Source: three-view drawing plus pictorial views. Frame: mm from the lowest corner of the part. A direction names the side the tool comes from. Coordinates: 2 decimals unless noted, no trailing zeros. Write each loop counter-clockwise with the first axis right and the second up, starting at its lowest first coordinate (ties: lowest second). Pieces come first, ordered by that corner, then holes. Notation, with made-up numbers: (69.25, 77.5) -> (73.25, 77.5) arc R22 ccw to (73.25, 91.5) -> close; hole circle Ø3 at (73, 22.25). An arc over 180 degrees is marked (long way). Write item = value, one per line.
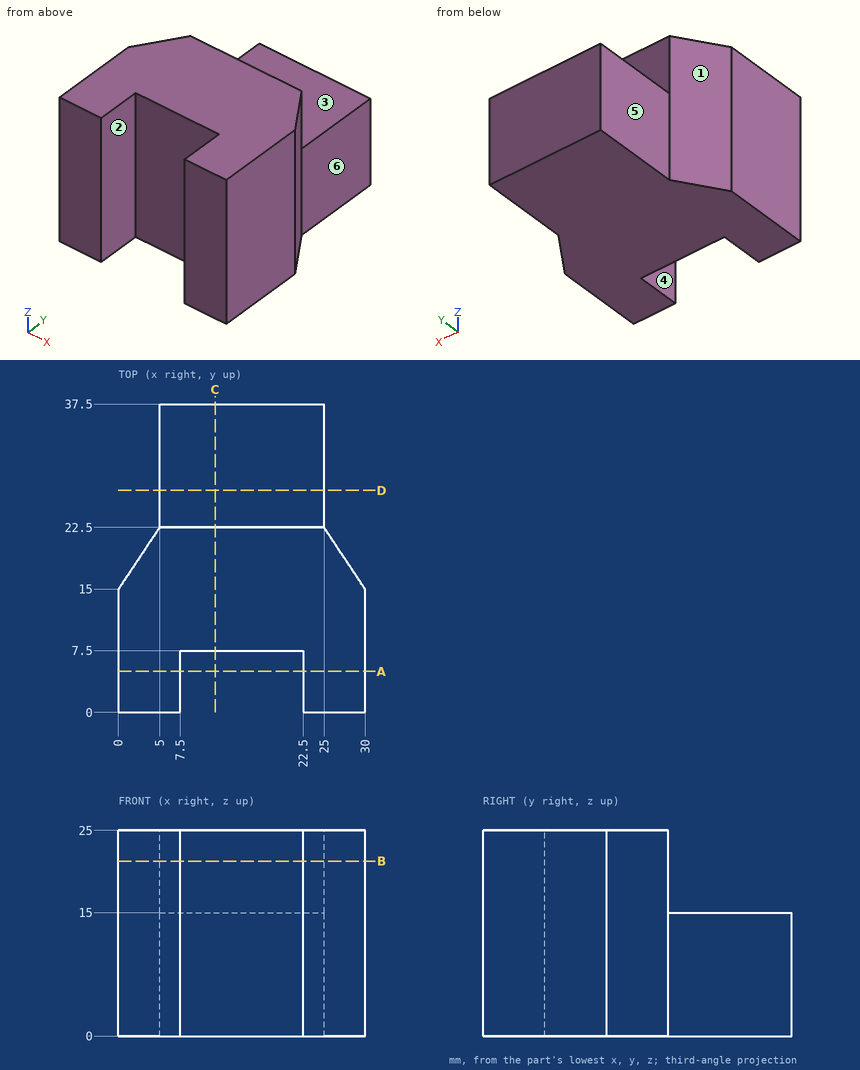
1) Cut plane B-B, the plane z = 21.25. Output: boundary loops of the cut face in (x, y).
Answer block:
outline = (0, 0) -> (7.5, 0) -> (7.5, 7.5) -> (22.5, 7.5) -> (22.5, 0) -> (30, 0) -> (30, 15) -> (25, 22.5) -> (5, 22.5) -> (0, 15) -> close
2) Cut plane C-C, the plane x = 11.75. Output: boundary loops of the cut face in (y, z), and give its area (3 significant figures).
Answer block:
outline = (7.5, 0) -> (37.5, 0) -> (37.5, 15) -> (22.5, 15) -> (22.5, 25) -> (7.5, 25) -> close
area = 600 mm2
3) First-contact query: pin 1 Ø6 at (x, z) = (16.5, 16) entering from -Y; pin 2 Ø7.5 at (y, z) = (30, 10) entering from +X; pin 3 Ø4.5 at (x, y) = (12.5, 31.5) entering from +Z. Flat tips, straight axial feed; report the tip coordinate or a pass-through.
Answer block:
pin_1 = 7.5
pin_2 = 25
pin_3 = 15
4) Cut plane D-D, the plane y = 27. Output: boundary loops of the cut face in (x, z).
Answer block:
outline = (5, 0) -> (25, 0) -> (25, 15) -> (5, 15) -> close
5) Cut plane A-A, the plane y = 5. Output: boundary loops of the cut face in (x, z).
Answer block:
outline = (0, 0) -> (7.5, 0) -> (7.5, 25) -> (0, 25) -> close; (22.5, 0) -> (30, 0) -> (30, 25) -> (22.5, 25) -> close
6) Pull-direction query (X, two-part tool) for the marked faces 1, 2 and 3; classes: +X half, -X half, draft (parallel to the pull), parting line (faces both ways), or undercut.
Answer block:
face_1 = -X half
face_2 = undercut
face_3 = draft
7) Material intervals for probe 1 along Y at (x, z) = (11.5, 18); probe 2 along X at (y, z) = (27, 4); probe 3 along Y at (x, z) = (9.75, 14.25), sorted ascending. Write a range as [from, to].
Answer block:
probe_1 = [7.5, 22.5]
probe_2 = [5, 25]
probe_3 = [7.5, 37.5]
8) Reachability of the marked faces 4, 5 and 6 from +Z, -Z, +X, -X, +Y, -Y: full face, straight path, thin tool, end or side. Return the list, or none.
Answer block:
face_4 = +Z, -Z, -Y
face_5 = +Z, -Z, -X, +Y
face_6 = +Z, -Z, +X, +Y
